The listing builds one solid part. Answer for the finished solid, in the listing's coordinates (mm). Face numbers are marked on the shaded views. Coordinates: 2 decimals unless noted, no trailing zeros. Order: outer loops, then holes, each group sorted by start corner. A loop starts at its lowest first (then second) coordinate and runs counter-clockwise, first axis right, second up. Notation, with made-up numbers: (-24, 88) -> (-8, 88) arc R24 ccw to (-8, 100) -> close; hole circle Ø6 at (5, -4). An arc over 180 degrees is marked (long way). Return JSON: item names as keys, results as strings.
from build123d import *

# Parameters (mm, degrees)
SKETCH1_W           = 250
SKETCH1_H           = 100
BOSS_EXTRUDE1_DEPTH = 5
CHAMFER2_SIZE       = 50
FILLET1_R           = 5
SKETCH2_W           = 8
SKETCH2_H           = 20
BOSS_EXTRUDE2_DEPTH = 35
SKETCH4_R           = 5
CUT_EXTRUDE1_DEPTH  = 184.643676722
FILLET2_R           = 10


with BuildPart() as part:
    # Sketch1 → Boss-Extrude1 (new body)
    with BuildSketch(Plane(origin=(0, 0, 0), x_dir=(1, 0, 0), z_dir=(0, 1, 0))):
        with Locations((-125, 50)):
            Rectangle(SKETCH1_W, SKETCH1_H)
    extrude(amount=BOSS_EXTRUDE1_DEPTH)

    # Chamfer2
    chamfer2_edges = [part.edges().sort_by_distance(p)[0] for p in [
        (0, 2.5, 0),
        (-250, 2.5, 0),
    ]]
    chamfer(chamfer2_edges, length=CHAMFER2_SIZE)

    # Fillet1
    fillet1_edges = [part.edges().sort_by_distance(p)[0] for p in [
        (-125, 5, -100),
    ]]
    fillet(fillet1_edges, radius=FILLET1_R - 0.0001)  # a hair under: the kernel refuses the full size

    # Sketch2 → Boss-Extrude2 (add)
    with BuildSketch(Plane.XZ):
        with Locations((-146, -10)):
            Rectangle(SKETCH2_W, SKETCH2_H)
        with Locations((-104, -10)):
            Rectangle(SKETCH2_W, SKETCH2_H)
    extrude(amount=BOSS_EXTRUDE2_DEPTH)

    # Sketch4 → Cut-Extrude1 (cut, through all)
    with BuildSketch(Plane(origin=(-100, 0, 0), x_dir=(0, 0, -1), z_dir=(1, 0, 0))):
        with Locations((10, -25)):
            Circle(SKETCH4_R)
    extrude(amount=-CUT_EXTRUDE1_DEPTH, mode=Mode.SUBTRACT)

    # Fillet2
    fillet2_edges = [part.edges().sort_by_distance(p)[0] for p in [
        (-104, -35, -20),
        (-146, -35, -20),
        (-146, -35, 0),
        (-104, -35, 0),
    ]]
    fillet(fillet2_edges, radius=FILLET2_R - 0.0001)  # a hair under: the kernel refuses the full size


solid = part.part
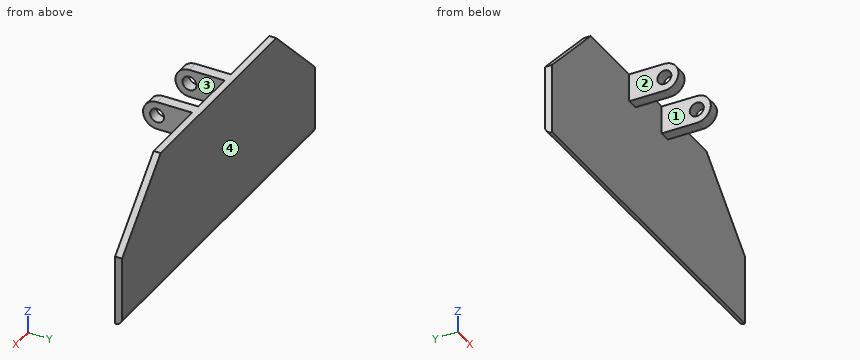
1. The part is cut by section A-A on y = -17.5. Give the vertices of the cut face in (x, z).
Answer block:
{"outline": "(-150, -20) -> (-142, -20) -> (-142, 0) -> (-150, 0) -> close; (-108, -20) -> (-100, -20) -> (-100, 0) -> (-108, 0) -> close"}
2. Each of these flat-tipped pins is pushed along its axis until it touches: pin 1 Ø6 at (y, z) = (-10, -12) entering from +X; pin 2 Ø12 at (x, z) = (-152.5, -43) entering from -Y; pin 3 Ø9 at (x, y) = (-147.5, -6.5) entering from -Z. Where does it stop, or does it pass through?
Answer block:
{"pin 1": "stops at x = -100", "pin 2": "stops at y = 0", "pin 3": "stops at z = -20"}
3. Consider line 1 (Y direction, x = -106, z = -10); line 2 (Y direction, x = -50.5, z = -60.5). Determine where each line is inside the solid, lowest interval first. Write a range as from..to.
Answer block:
{"line 1": "y = -35..-30, -20..5", "line 2": "y = 0..5"}
4. Determine the mould class of the marked faces 1, 2, 3 and 4 for opening direction X: pulls with the +X half, pulls with the -X half, needs draft (parallel to the pull), parting line crosses it, or undercut.
Answer block:
{"face 1": "undercut", "face 2": "pulls with the -X half", "face 3": "undercut", "face 4": "needs draft"}
5. The part is cut by section C-C on z = -39. Give the vertices of the cut face in (x, y).
Answer block:
{"outline": "(-239, 0) -> (-11, 0) -> (-11, 5) -> (-239, 5) -> close"}
